For this review, take the finished solid that the model builds, in its own axes (mm). A direction names the side the tool comes from. Coordinates: 2 decimals unless noted, no trailing zeros. Write each loop counter-clockwise with the first axis right and the second up, starting at its lowest first coordinate (ties: lowest second). Pieces come first, ordered by that corner, then holes.
```python
from build123d import *

# Parameters (mm, degrees)
F0_W     = 39.5
F0_H     = 155
F1_DEPTH = 9.7
F2_R     = 11
F3_R     = 11
F4_DEPTH = 9.701
F5_R     = 5.25
F6_DEPTH = 6


with BuildPart() as f1:
    # F0 (on Top) → F1 (new body)
    with BuildSketch(Plane.XY):
        Rectangle(F0_W, F0_H)
    extrude(amount=F1_DEPTH)

    # F2
    f2_edges = [f1.edges().sort_by_distance(p)[0] for p in [
        (-19.75, 77.5, 4.85),
        (19.75, 77.5, 4.85),
        (19.75, -77.5, 4.85),
        (-19.75, -77.5, 4.85),
    ]]
    fillet(f2_edges, radius=F2_R)

    # F3 (on face) → F4 (cut, through all)
    with BuildSketch(Plane.XY.offset(9.7)):
        with Locations((0, -57.5)):
            Circle(F3_R)
    extrude(amount=-F4_DEPTH, mode=Mode.SUBTRACT)

    # F5 (on face) → F6 (join)
    with BuildSketch(Plane.XY.offset(9.7)):
        with Locations((0, 59)):
            Circle(F5_R)
    extrude(amount=F6_DEPTH)


solid = f1.part
```
Q1. Add section A-A (x = 0). State the section outline as (y, z) points, then the cut area to 3 significant figures.
Ans:
outline: (-77.5, 0) - (-68.5, 0) - (-68.5, 9.7) - (-77.5, 9.7) - close; (-46.5, 0) - (77.5, 0) - (77.5, 9.7) - (64.25, 9.7) - (64.25, 15.7) - (53.75, 15.7) - (53.75, 9.7) - (-46.5, 9.7) - close
area: 1,350 mm2
Q2. Tool access review of faces 4 (the flat face through (19.75, -1, 5)), 5 (the cylindrical face through (-1.138, 53.875, 12.658)): name each direction out of +Z, -Z, +X, -X, +Y, -Y from which nothing blocks a thin tool from reaching the whole face with its end or side.
Ans:
face 4: +Z, -Z, +X, +Y, -Y
face 5: +Z
Q3. For probe 1 along Y at (x, z) = (0, 6.25); probe 2 along Z at (x, y) = (-12, -0.5); probe 3 along X at (y, z) = (-66.5, 4.25), list the stretches that pass through material, from the lowest coordinate up.
Ans:
probe 1: y = -77.5 to -68.5, -46.5 to 77.5
probe 2: z = 0 to 9.7
probe 3: x = -19.75 to -6.32, 6.32 to 19.75
Q4. Add section C-C (y = -57.5). State the section outline as (x, z) points, then the cut area to 3 significant figures.
Ans:
outline: (-19.75, 0) - (-11, 0) - (-11, 9.7) - (-19.75, 9.7) - close; (11, 0) - (19.75, 0) - (19.75, 9.7) - (11, 9.7) - close
area: 170 mm2
Q5. Add section B-B (z = 6). State the section outline as (x, y) points, then the cut area to 3 significant figures.
Ans:
outline: (-19.75, -66.5) arc R11 ccw to (-8.75, -77.5) - (8.75, -77.5) arc R11 ccw to (19.75, -66.5) - (19.75, 66.5) arc R11 ccw to (8.75, 77.5) - (-8.75, 77.5) arc R11 ccw to (-19.75, 66.5) - close; hole circle Ø22 at (0, -57.5)
area: 5,640 mm2
Q6. Clearance check with flat-ended pins moving along their axes: pin 1 Ø17.5 at (x, y) = (0, -57.5) entering from -Z; pin 2 Ø2 at (x, z) = (15.5, 2) entering from +Y; pin 3 Ø20 at (x, y) = (-7, 30) entering from +Z. State where each tip first meets the part, or that it passes through.
Ans:
pin 1: passes through
pin 2: stops at y = 75.88
pin 3: stops at z = 9.7
Q7. Draft analysis for pull direction Y (two halves, no side actions). For faces 1 (the cylindrical face through (-1.432, -46.594, 4.918)), 2 (the flat face through (0, 77.5, 5)), 3 (the flat face through (0, 1, 0)), state which applies: +Y half, -Y half, draft (parallel to the pull), parting line (faces both ways), or undercut.
Ans:
face 1: undercut
face 2: +Y half
face 3: draft
Q8. Add section D-D (y = 59). State the section outline as (x, z) points.
Ans:
outline: (-19.75, 0) - (19.75, 0) - (19.75, 9.7) - (5.25, 9.7) - (5.25, 15.7) - (-5.25, 15.7) - (-5.25, 9.7) - (-19.75, 9.7) - close
